Input: part model. Units: mm. Frame: model coordinates. Round coordinates to 2 decimals unless told otherwise and drop trailing zeros. Use one line per item in the form item = value.
```python
from build123d import *

# Parameters (mm, degrees)
SKETCH1_R      = 2.1
EXTRUDE1_DEPTH = 304.8


with BuildPart() as part:
    # Sketch1 → Extrude1 (new, symmetric)
    with BuildSketch(Plane.XY):
        with BuildLine():
            Line((-3.900660172, 0), (-3.900660172, -2.84))
            Line((-3.900660172, -2.84), (-6.56, -5.499339828))
            Line((-6.56, -5.499339828), (-8.2, -5.499339828))
            Line((-8.2, -5.499339828), (-8.2, -2.84))
            Line((-8.2, -2.84), (-10, -4.64))
            Line((-10, -4.64), (-10, -8.2))
            ThreePointArc((-10, -8.2), (-9.472792206, -9.472792206), (-8.2, -10))
            Line((-8.2, -10), (-4.64, -10))
            Line((-4.64, -10), (-2.84, -8.2))
            Line((-2.84, -8.2), (-5.499339828, -8.2))
            Line((-5.499339828, -8.2), (-5.499339828, -6.56))
            Line((-5.499339828, -6.56), (-2.84, -3.900660172))
            Line((-2.84, -3.900660172), (0, -3.900660172))
            Line((0, -3.900660172), (2.84, -3.900660172))
            Line((2.84, -3.900660172), (5.499339828, -6.56))
            Line((5.499339828, -6.56), (5.499339828, -8.2))
            Line((5.499339828, -8.2), (2.84, -8.2))
            Line((2.84, -8.2), (4.64, -10))
            Line((4.64, -10), (8.2, -10))
            ThreePointArc((8.2, -10), (9.472792206, -9.472792206), (10, -8.2))
            Line((10, -8.2), (10, -4.64))
            Line((10, -4.64), (8.2, -2.84))
            Line((8.2, -2.84), (8.2, -5.499339828))
            Line((8.2, -5.499339828), (6.56, -5.499339828))
            Line((6.56, -5.499339828), (3.900660172, -2.84))
            Line((3.900660172, -2.84), (3.900660172, 0))
            Line((3.900660172, 0), (3.900660172, 2.84))
            Line((3.900660172, 2.84), (6.56, 5.499339828))
            Line((6.56, 5.499339828), (8.2, 5.499339828))
            Line((8.2, 5.499339828), (8.2, 2.84))
            Line((8.2, 2.84), (10, 4.64))
            Line((10, 4.64), (10, 8.2))
            ThreePointArc((10, 8.2), (9.472792206, 9.472792206), (8.2, 10))
            Line((8.2, 10), (4.64, 10))
            Line((4.64, 10), (2.84, 8.2))
            Line((2.84, 8.2), (5.499339828, 8.2))
            Line((5.499339828, 8.2), (5.499339828, 6.56))
            Line((5.499339828, 6.56), (2.84, 3.900660172))
            Line((2.84, 3.900660172), (0, 3.900660172))
            Line((0, 3.900660172), (-2.84, 3.900660172))
            Line((-2.84, 3.900660172), (-5.499339828, 6.56))
            Line((-5.499339828, 6.56), (-5.499339828, 8.2))
            Line((-5.499339828, 8.2), (-2.84, 8.2))
            Line((-2.84, 8.2), (-4.64, 10))
            Line((-4.64, 10), (-8.2, 10))
            ThreePointArc((-8.2, 10), (-9.472792206, 9.472792206), (-10, 8.2))
            Line((-10, 8.2), (-10, 4.64))
            Line((-10, 4.64), (-8.2, 2.84))
            Line((-8.2, 2.84), (-8.2, 5.499339828))
            Line((-8.2, 5.499339828), (-6.56, 5.499339828))
            Line((-6.56, 5.499339828), (-3.900660172, 2.84))
            Line((-3.900660172, 2.84), (-3.900660172, 0))
        make_face()
        with Locations(Location((0, 0, 0), (0, 0, 180))):
            Circle(SKETCH1_R, mode=Mode.SUBTRACT)
        Polygon((-8.2, -8.2), (-8.2, -6.569339828), (-7.63, -6.569339828), (-6.569339828, -7.63), (-6.569339828, -8.2), align=None, mode=Mode.SUBTRACT)
        Polygon((-8.2, 6.569339828), (-8.2, 8.2), (-6.569339828, 8.2), (-6.569339828, 7.63), (-7.63, 6.569339828), align=None, mode=Mode.SUBTRACT)
        Polygon((6.569339828, 8.2), (8.2, 8.2), (8.2, 6.569339828), (7.63, 6.569339828), (6.569339828, 7.63), align=None, mode=Mode.SUBTRACT)
        Polygon((8.2, -6.569339828), (8.2, -8.2), (6.569339828, -8.2), (6.569339828, -7.63), (7.63, -6.569339828), align=None, mode=Mode.SUBTRACT)
    extrude(amount=EXTRUDE1_DEPTH, both=True)


solid = part.part
```
(1) First-contact query: pin 1 Ø8 at (y, z) = (-3.5, -108) entering from +X; pin 2 Ø1.5 at (y, z) = (-0.5, 155) entering from -X; pin 3 Ø1.7 at (y, z) = (0.5, 134.5) entering from +X; pin 4 Ø2 at (x, y) = (2, -6.5) entering from +Z. Flat tips, straight axial feed; report the tip coordinate or a pass-through.
Derived:
pin_1 = 10
pin_2 = -3.9
pin_3 = 3.9
pin_4 = through
(2) Material intervals for L1, parallel to Y at x = 0, z = -155.5; L2, parallel to X at y = 5, z = -252; L3, parallel to X at y = -3, z = 269, sorted ascending.
Derived:
L1 = -3.9 to -2.1, 2.1 to 3.9
L2 = -10 to -8.2, -6.06 to -3.94, 3.94 to 6.06, 8.2 to 10
L3 = -8.36 to -8.2, -4.06 to 4.06, 8.2 to 8.36
(3) Cut plane A-A on z = 47. Count the separate pieces of the cut face and the enclosed holes in it, then the cut area to 3 significant figures.
Derived:
separate_pieces = 1
enclosed_holes = 5
area = 160 mm^2
